Input: part model. Units: mm. Frame: model coordinates. Face numbers are marked on the shaded views. A direction names the side the tool comes from. Give positions to 0.01 mm unless a question says otherwise; leave off trailing zeros. Write each loop counter-clockwise with the first axis right and the second up, starting at its lowest first coordinate (ties: lowest second). Pieces come first, ordered by that corner, then holes.
```python
from build123d import *

# Parameters (mm, degrees)
F0_R     = 1.5
F0_R_2   = 2
F0_R_3   = 14.5
F1_DEPTH = 4
F2_R     = 12
F0_R_4   = 12.4
F3_DEPTH = 6
F4_DEPTH = 16


with BuildPart() as f1:
    # F0 (on Top) → F1 (new body)
    with BuildSketch(Plane.XY):
        with BuildLine():
            Line((40.1261364576, -50), (50, -50))
            Line((50, -50), (50, -40.1261364576))
            ThreePointArc((50, -40.1261364576), (48.5323223277, -39.658202653), (47, -39.5))
            Line((47, -39.5), (47, -47))
            Line((47, -47), (39.5, -47))
            ThreePointArc((39.5, -47), (39.658202653, -48.5323223277), (40.1261364576, -50))
        make_face()
        with BuildLine():
            Line((-40.1261364576, -50), (40.1261364576, -50))
            ThreePointArc((40.1261364576, -50), (39.658202653, -48.5323223277), (39.5, -47))
            Line((39.5, -47), (-39.5, -47))
            ThreePointArc((-39.5, -47), (-39.658202653, -48.5323223277), (-40.1261364576, -50))
        make_face()
        with BuildLine():
            ThreePointArc((47, -39.5), (48.5323223277, -39.658202653), (50, -40.1261364576))
            Line((50, -40.1261364576), (50, 40.1261364576))
            ThreePointArc((50, 40.1261364576), (48.5323223277, 39.658202653), (47, 39.5))
            Line((47, 39.5), (47, -39.5))
        make_face()
        with BuildLine():
            Line((-50, -50), (-40.1261364576, -50))
            ThreePointArc((-40.1261364576, -50), (-39.658202653, -48.5323223277), (-39.5, -47))
            Line((-39.5, -47), (-47, -47))
            Line((-47, -47), (-47, -39.5))
            ThreePointArc((-47, -39.5), (-52.0432569895, -41.4488236438), (-54.4656023889, -46.2825176166))
            ThreePointArc((-54.4656023889, -46.2825176166), (-52.2758824324, -48.1930098751), (-50, -50))
        make_face()
        with BuildLine():
            ThreePointArc((47, -39.5), (41.6966991411, -41.6966991411), (39.5, -47))
            Line((39.5, -47), (47, -47))
            Line((47, -47), (47, -39.5))
        make_face()
        with Locations((44, -44)):
            Circle(F0_R, mode=Mode.SUBTRACT)
        with BuildLine():
            Line((-39.5, -47), (39.5, -47))
            ThreePointArc((39.5, -47), (41.6966991411, -41.6966991411), (47, -39.5))
            Line((47, -39.5), (47, 39.5))
            ThreePointArc((47, 39.5), (41.6966991411, 41.6966991411), (39.5, 47))
            Line((39.5, 47), (-39.5, 47))
            ThreePointArc((-39.5, 47), (-41.6966991411, 41.6966991411), (-47, 39.5))
            Line((-47, 39.5), (-47, -39.5))
            ThreePointArc((-47, -39.5), (-41.6966991411, -41.6966991411), (-39.5, -47))
        make_face()
        with Locations((-28.9172229711, -9)):
            Circle(F0_R_2, mode=Mode.SUBTRACT)
        with Locations((-28.9172229711, 9)):
            Circle(F0_R_2, mode=Mode.SUBTRACT)
        Circle(F0_R_3, mode=Mode.SUBTRACT)
        with BuildLine():
            ThreePointArc((47, 39.5), (48.5323223277, 39.658202653), (50, 40.1261364576))
            Line((50, 40.1261364576), (50, 50))
            Line((50, 50), (40.1261364576, 50))
            ThreePointArc((40.1261364576, 50), (39.658202653, 48.5323223277), (39.5, 47))
            Line((39.5, 47), (47, 47))
            Line((47, 47), (47, 39.5))
        make_face()
        with BuildLine():
            ThreePointArc((-74.8632505062, 0), (-69.5376936802, -25.2890069281), (-54.4656023889, -46.2825176166))
            ThreePointArc((-54.4656023889, -46.2825176166), (-52.0432569895, -41.4488236438), (-47, -39.5))
            Line((-47, -39.5), (-47, 39.5))
            ThreePointArc((-47, 39.5), (-52.0432569895, 41.4488236438), (-54.4656023889, 46.2825176166))
            ThreePointArc((-54.4656023889, 46.2825176166), (-69.5376936802, 25.2890069281), (-74.8632505062, 0))
        make_face()
        with Locations((-62.4172229711, -9)):
            Circle(F0_R_2, mode=Mode.SUBTRACT)
        with Locations((-62.4172229711, 9)):
            Circle(F0_R_2, mode=Mode.SUBTRACT)
        with BuildLine():
            ThreePointArc((-47.3632505062, 0), (-54.8632505062, -7.5), (-62.3632505062, 0))
            ThreePointArc((-62.3632505062, 0), (-54.8632505062, 7.5), (-47.3632505062, 0))
        make_face(mode=Mode.SUBTRACT)
        with BuildLine():
            Line((-47, -47), (-39.5, -47))
            ThreePointArc((-39.5, -47), (-41.6966991411, -41.6966991411), (-47, -39.5))
            Line((-47, -39.5), (-47, -47))
        make_face()
        with Locations((-44, -44)):
            Circle(F0_R, mode=Mode.SUBTRACT)
        with BuildLine():
            ThreePointArc((39.5, 47), (41.6966991411, 41.6966991411), (47, 39.5))
            Line((47, 39.5), (47, 47))
            Line((47, 47), (39.5, 47))
        make_face()
        with Locations((44, 44)):
            Circle(F0_R, mode=Mode.SUBTRACT)
        with BuildLine():
            ThreePointArc((39.5, 47), (39.658202653, 48.5323223277), (40.1261364576, 50))
            Line((40.1261364576, 50), (-40.1261364576, 50))
            ThreePointArc((-40.1261364576, 50), (-39.658202653, 48.5323223277), (-39.5, 47))
            Line((-39.5, 47), (39.5, 47))
        make_face()
        with BuildLine():
            ThreePointArc((-54.4656023889, 46.2825176166), (-52.0432569895, 41.4488236438), (-47, 39.5))
            Line((-47, 39.5), (-47, 47))
            Line((-47, 47), (-39.5, 47))
            ThreePointArc((-39.5, 47), (-39.658202653, 48.5323223277), (-40.1261364576, 50))
            Line((-40.1261364576, 50), (-50, 50))
            ThreePointArc((-50, 50), (-52.2758824324, 48.1930098751), (-54.4656023889, 46.2825176166))
        make_face()
        with BuildLine():
            Line((-47, 47), (-47, 39.5))
            ThreePointArc((-47, 39.5), (-41.6966991411, 41.6966991411), (-39.5, 47))
            Line((-39.5, 47), (-47, 47))
        make_face()
        with Locations((-44, 44)):
            Circle(F0_R, mode=Mode.SUBTRACT)
    extrude(amount=F1_DEPTH)

    # F2
    f2_edges = [f1.edges().sort_by_distance(p)[0] for p in [
        (-50, 50, 2),
        (50, 50, 2),
        (50, -50, 2),
        (-50, -50, 2),
    ]]
    fillet(f2_edges, radius=F2_R)

    # F0 (on Top) → F3 (join)
    with BuildSketch(Plane.XY):
        Circle(F0_R_3)
        Circle(F0_R_4, mode=Mode.SUBTRACT)
    extrude(amount=F3_DEPTH)

    # F0 (on Top) → F4 (join)
    with BuildSketch(Plane.XY):
        Circle(F0_R_4)
    extrude(amount=F4_DEPTH)


solid = f1.part
```
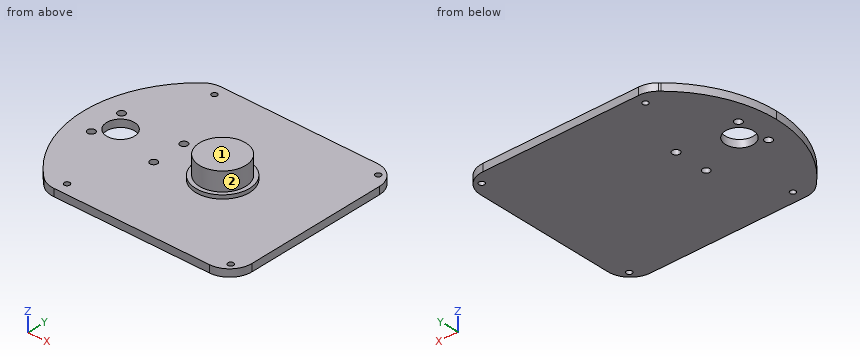
Item 1: Ray query, line 1 (Y direction, x = -44, z = 1.15); line 2 (Y direction, x = -29, z = 3.75); line 3 (Z direction, x = 3, y = 27). Return the intervals inside material, ascending.
Item 2: Section B-B (y = 4.5). Return loops of the section in (x, z).
Item 3: Section C-C (x = 0). Return loops of the section in (y, z).
Item 4: Section D-D (y = -9). Return loops of the section in (x, z), and give its area (3 significant figures).
Item 5: Set-up query: the marked faces 1 and 2. Return all of +Z, -Z, +X, -X, +Y, -Y with unobstructed straight access to the full face (end or side cutting, diameter ignored); none if empty.
Item 6: Pin query (flat end, axial travel): pin 1 (2.5 mm diameter, centred on x = -28.92, y = -9, fed in from +Z); pin 2 (8 mm diameter, centred on x = -12, z = 10.5, fed in from -Y); pin 3 (3.5 mm diameter, centred on x = -44, y = 44, fed in from +Z); pin 4 (1.5 mm diameter, centred on x = 5, z = 8.5, fed in from +Y). Return the tip coordinate at first contact, or that it passes through.
Item 7: Section A-A (z = 2). Give the number of separate pieces and of enclosed holes in the cut face, and give its area (3 significant figures).
Solved:
1. line 1: y = -50 to -45.5, -42.5 to 42.5, 45.5 to 50
1. line 2: y = -50 to -11, -7 to 7, 11 to 50
1. line 3: z = 0 to 4
2. outline: (-74.7, 0) - (-60.86, 0) - (-60.86, 4) - (-74.7, 4) - close; (-48.86, 0) - (50, 0) - (50, 4) - (13.78, 4) - (13.78, 6) - (11.55, 6) - (11.55, 16) - (-11.55, 16) - (-11.55, 6) - (-13.78, 6) - (-13.78, 4) - (-48.86, 4) - close
3. outline: (-50, 0) - (50, 0) - (50, 4) - (14.5, 4) - (14.5, 6) - (12.4, 6) - (12.4, 16) - (-12.4, 16) - (-12.4, 6) - (-14.5, 6) - (-14.5, 4) - (-50, 4) - close
4. outline: (-74.21, 0) - (-64.42, 0) - (-64.42, 4) - (-74.21, 4) - close; (-60.42, 0) - (-30.92, 0) - (-30.92, 4) - (-60.42, 4) - close; (-26.92, 0) - (50, 0) - (50, 4) - (11.37, 4) - (11.37, 6) - (8.53, 6) - (8.53, 16) - (-8.53, 16) - (-8.53, 6) - (-11.37, 6) - (-11.37, 4) - (-26.92, 4) - close
4. area: 681 mm2
5. face 1: +Z, +X, -X, +Y, -Y
5. face 2: +Z
6. pin 1: passes through
6. pin 2: stops at y = -9.47
6. pin 3: stops at z = 4
6. pin 4: stops at y = 11.65
7. separate pieces: 1
7. enclosed holes: 9
7. area: 11,400 mm2
